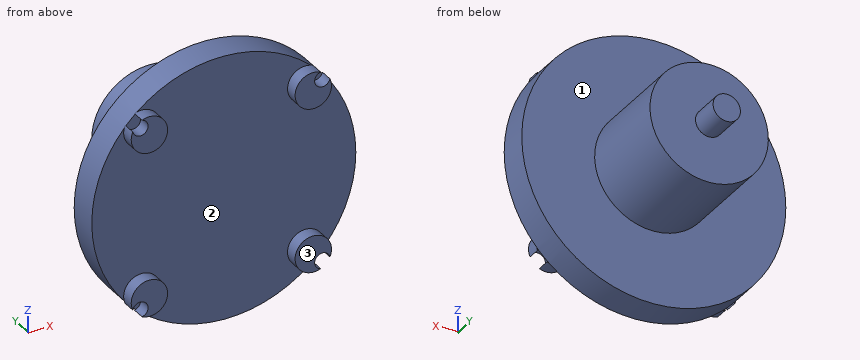
from build123d import *

# Parameters (mm, degrees)
SKETCH1_R           = 58
BOSS_EXTRUDE1_DEPTH = 14
SKETCH2_R           = 8
BOSS_EXTRUDE2_DEPTH = 6
SKETCH3_R           = 26
BOSS_EXTRUDE3_DEPTH = 58
SKETCH4_R           = 6
BOSS_EXTRUDE4_DEPTH = 72
SKETCH5_R           = 3.4
CUT_EXTRUDE1_DEPTH  = 110.142109197


with BuildPart() as part:
    # Sketch1 → Boss-Extrude1 (new body)
    with BuildSketch(Plane(origin=(0, 0, 0), x_dir=(1, 0, 0), z_dir=(0, 1, 0))):
        with Locations(Location((0, 0, 0), (0, 0, 270))):
            Circle(SKETCH1_R)
    extrude(amount=BOSS_EXTRUDE1_DEPTH)

    # Sketch2 → Boss-Extrude2 (add)
    with BuildSketch(Plane(origin=(0, 0, 0), x_dir=(1, 0, 0), z_dir=(0, 1, 0))):
        with Locations(Location((-36, -36, 0), (0, 0, 270))):
            Circle(SKETCH2_R)
        with Locations(Location((36, -36, 0), (0, 0, 270))):
            Circle(SKETCH2_R)
        with Locations(Location((-36, 36, 0), (0, 0, 270))):
            Circle(SKETCH2_R)
        with Locations(Location((36, 36, 0), (0, 0, 270))):
            Circle(SKETCH2_R)
    extrude(amount=-BOSS_EXTRUDE2_DEPTH)

    # Sketch3 → Boss-Extrude3 (add)
    with BuildSketch(Plane(origin=(0, 0, 0), x_dir=(1, 0, 0), z_dir=(0, 1, 0))):
        with Locations(Location((0, 0, 0), (0, 0, 90))):
            Circle(SKETCH3_R)
    extrude(amount=BOSS_EXTRUDE3_DEPTH)

    # Sketch4 → Boss-Extrude4 (add)
    with BuildSketch(Plane(origin=(0, 0, 0), x_dir=(1, 0, 0), z_dir=(0, 1, 0))):
        with Locations(Location((0, 0, 0), (0, 0, 270))):
            Circle(SKETCH4_R)
    extrude(amount=BOSS_EXTRUDE4_DEPTH)

    # Sketch5 → Cut-Extrude1 (cut, through all)
    with BuildSketch(Plane(origin=(0, 0, 0), x_dir=(1, 0, 0), z_dir=(0, 1, 0))):
        with Locations((-40, -40)):
            Circle(SKETCH5_R)
        with Locations((40, -40)):
            Circle(SKETCH5_R)
        with Locations((-40, 40)):
            Circle(SKETCH5_R)
        with Locations((40, 40)):
            Circle(SKETCH5_R)
    extrude(amount=-CUT_EXTRUDE1_DEPTH, mode=Mode.SUBTRACT)


solid = part.part
Check sheet for the modelled part. Datum: model origin and axes. Units: mm. Face numbers are marked on the shaded views. A direction names the side the tool comes from. Round coordinates to 2 decimals unless told otherwise and drop trailing zeros. Write each loop counter-clockwise with the first axis right and the second up, starting at its lowest first coordinate (ties: lowest second). Pieces come first, ordered by that corner, then holes. Notation, with made-up numbers: (-16, 19) - (34, 19) arc R31 ccw to (34, 55) - close; hole circle Ø5 at (-20, 60.25). An arc over 180 degrees is marked (long way). Return JSON: item names as keys, results as strings.
Q1. Scan lines: L1, parallel to Y at x = 23, z = -3; L2, parallel to Y at x = 39, z = -42.5; L3, parallel to X at y = -3.25, z = 40. Record each from-to range of solid material in increasing order. Write a range as from..to.
Returned:
{"L1": "y = 0..58", "L2": "y = 0..14", "L3": "x = -36.6..-29.07, 29.07..36.6"}
Q2. Cross-section at C-C (y = 34). Record the boundary of the cut face in (x, z), then the cut area to 3 significant figures.
Returned:
{"outline": "circle Ø52 at (0, 0)", "area": "2,120 mm²"}
Q3. Access from +Z, -Z, +X, -X, +Y, -Y to the whole of each face (thin tool, end or side, straight path). Record for the marked faces 1, 2 and 3.
Returned:
{"face 1": "+Y", "face 2": "-Y", "face 3": "+Z, -Z, +X, -X, -Y"}
Q4. Cross-section at D-D (x = 15.5). Record the boundary of the cut face in (y, z).
Returned:
{"outline": "(0, -55.89) - (14, -55.89) - (14, -20.87) - (58, -20.87) - (58, 20.87) - (14, 20.87) - (14, 55.89) - (0, 55.89) - close"}
Q5. Cross-section at A-A (z = 0). Record the boundary of the cut face in (x, y), then the cut area to 3 significant figures.
Returned:
{"outline": "(-58, 0) - (58, 0) - (58, 14) - (26, 14) - (26, 58) - (6, 58) - (6, 72) - (-6, 72) - (-6, 58) - (-26, 58) - (-26, 14) - (-58, 14) - close", "area": "4,080 mm²"}
Q6. Depth check by flat-ended pin: P1, Ø6, axis at x = -40, z = -40, coming from the +Y side; P2, Ø4, axis at x = 31, z = -2.5, coming from the -Y side; P3, Ø8, axis at y = 50.5, z = 21.5, coming from the +X side. Enter the tip coordinate at first touch or a pass-through.
Returned:
{"P1": "stops at y = 14", "P2": "stops at y = 0", "P3": "stops at x = 19.23"}
Q7. Cross-section at B-B (x = 0). Record the boundary of the cut face in (y, z), then the cut area to 3 significant figures.
Returned:
{"outline": "(0, -58) - (14, -58) - (14, -26) - (58, -26) - (58, -6) - (72, -6) - (72, 6) - (58, 6) - (58, 26) - (14, 26) - (14, 58) - (0, 58) - close", "area": "4,080 mm²"}
